```python
from build123d import *

# Parameters (mm, degrees)
SKETCH1_W           = 7.8
SKETCH1_H           = 1
BOSS_EXTRUDE1_DEPTH = 5
SKETCH2_W           = 7.465
SKETCH2_H           = 0.5
CUT_EXTRUDE1_DEPTH  = 0.5
SKETCH3_W           = 14.93
SKETCH3_H           = 0.5
CUT_EXTRUDE2_DEPTH  = 0.5
BOSS_EXTRUDE2_DEPTH = 0.5
SKETCH5_W           = 1
SKETCH5_H           = 2.195949596
BOSS_EXTRUDE3_DEPTH = 7.5
SKETCH6_W           = 0.2
SKETCH6_H           = 0.5
SKETCH6_W_2         = 0.5
SKETCH6_W_3         = 0.413933432
BOSS_EXTRUDE4_DEPTH = 0.5
SKETCH8_W           = 14.93
SKETCH8_H           = 0.5
CUT_EXTRUDE3_DEPTH  = 0.5
SKETCH9_W           = 14.93
SKETCH9_H           = 0.084331677
CUT_EXTRUDE4_DEPTH  = 0.5
SKETCH12_W          = 14.93
SKETCH12_H          = 1.2
CUT_EXTRUDE5_DEPTH  = 0.5


with BuildPart() as part:
    # Sketch1 → Boss-Extrude1 (new body)
    with BuildSketch(Plane(origin=(0, 0, 0), x_dir=(1, 0, 0), z_dir=(0, 1, 0))):
        with Locations((3.9, 15.43)):
            Rectangle(SKETCH1_W, SKETCH1_H)
        Polygon((7.8, 15.93), (8.8, 14.93), (7.8, 14.93), align=None)
        Polygon((7.8, -1), (7.8, 0), (7.8, 14.93), (8.8, 14.93), (8.8, 0), align=None)
        Polygon((-1, 0), (0, 0), (7.8, 0), (7.8, -1), (0, -1), align=None)
        Polygon((0, 15.93), (0, 14.93), (0, 0), (-1, 0), (-1, 14.93), align=None)
    extrude(amount=BOSS_EXTRUDE1_DEPTH)

    # Sketch2 → Cut-Extrude1 (cut)
    with BuildSketch(Plane(origin=(0, 0, 0), x_dir=(0, 0, -1), z_dir=(1, 0, 0))):
        with Locations((11.1975, 0.75)):
            Rectangle(SKETCH2_W, SKETCH2_H)
        with Locations((3.7325, 0.75)):
            Rectangle(SKETCH2_W, SKETCH2_H)
    extrude(amount=-CUT_EXTRUDE1_DEPTH, mode=Mode.SUBTRACT)

    # Sketch3 → Cut-Extrude2 (cut)
    with BuildSketch(Plane.ZY.offset(-7.8)):
        with Locations((-7.465, 0.75)):
            Rectangle(SKETCH3_W, SKETCH3_H)
    extrude(amount=-CUT_EXTRUDE2_DEPTH, mode=Mode.SUBTRACT)

    # Sketch4 → Boss-Extrude2 (add)
    with BuildSketch(Plane(origin=(0, 5, 0), x_dir=(1, 0, 0), z_dir=(0, 1, 0))):
        Polygon((-1, 0), (0, -1), (7.8, -1), (8.8, 0), (8.8, 14.93), (7.8, 15.93), (0, 15.93), (-1, 14.93), align=None)
    extrude(amount=BOSS_EXTRUDE2_DEPTH)

    # Sketch5 → Boss-Extrude3 (add)
    with BuildSketch(Plane.XZ.offset(-5)):
        with Locations((4.4, -12.832025202)):
            Rectangle(SKETCH5_W, SKETCH5_H)
        with Locations((3.4, -12.832025202)):
            Rectangle(SKETCH5_W, SKETCH5_H)
        with Locations((3.4, -10.636075606)):
            Rectangle(SKETCH5_W, SKETCH5_H)
        with Locations((4.4, -10.636075606)):
            Rectangle(SKETCH5_W, SKETCH5_H)
    extrude(amount=BOSS_EXTRUDE3_DEPTH)

    # Sketch6 → Boss-Extrude4 (add)
    with BuildSketch(Plane.XZ.offset(2.5)):
        with Locations((4, -10.984050404)):
            Rectangle(SKETCH6_W, SKETCH6_H)
        with Locations((3.8, -10.984050404)):
            Rectangle(SKETCH6_W, SKETCH6_H)
        with Locations((3.8, -11.484050404)):
            Rectangle(SKETCH6_W, SKETCH6_H)
        with Locations((4, -11.484050404)):
            Rectangle(SKETCH6_W, SKETCH6_H)
        with Locations((4.35, -11.484050404)):
            Rectangle(SKETCH6_W_2, SKETCH6_H)
        with Locations((4.35, -11.984050404)):
            Rectangle(SKETCH6_W_2, SKETCH6_H)
        Polygon((3.9, -11.734050404), (3.7, -11.734050404), (3.7, -12.234050404), (3.986066568, -12.234050404), (4.1, -12.234050404), (4.1, -11.734050404), align=None)
        with Locations((3.493033284, -11.484050404)):
            Rectangle(SKETCH6_W_3, SKETCH6_H)
        with Locations((3.493033284, -11.984050404)):
            Rectangle(SKETCH6_W_3, SKETCH6_H)
        Polygon((3.986066568, -12.234050404), (3.7, -12.234050404), (3.7, -12.768693535), (4.1, -12.768693535), (4.1, -12.234050404), align=None)
    extrude(amount=BOSS_EXTRUDE4_DEPTH)

    # Sketch8 → Cut-Extrude3 (cut)
    with BuildSketch(Plane.ZY.offset(-7.8)):
        with Locations((-7.465, 1.334331677)):
            Rectangle(SKETCH8_W, SKETCH8_H)
    extrude(amount=-CUT_EXTRUDE3_DEPTH, mode=Mode.SUBTRACT)

    # Sketch9 → Cut-Extrude4 (cut)
    with BuildSketch(Plane.ZY.offset(-7.8)):
        with Locations((-7.465, 1.042165838)):
            Rectangle(SKETCH9_W, SKETCH9_H)
    extrude(amount=-CUT_EXTRUDE4_DEPTH, mode=Mode.SUBTRACT)

    # Sketch12 → Cut-Extrude5 (cut)
    with BuildSketch(Plane(origin=(0, 0, 0), x_dir=(0, 0, -1), z_dir=(1, 0, 0))):
        with Locations((7.465, 1.6)):
            Rectangle(SKETCH12_W, SKETCH12_H)
    extrude(amount=-CUT_EXTRUDE5_DEPTH, mode=Mode.SUBTRACT)


solid = part.part
```
Verification items for the finished model (mm, model axes). A direction names the side the tool comes from. Coordinates: 2 decimals unless noted, no trailing zeros. Order: outer loops, then holes, each group sorted by start corner. A loop starts at its lowest first (then second) coordinate and runs counter-clockwise, first axis right, second up. Notation, with made-up numbers: (16.5, 41) -> (59.5, 41) arc R20 cw to (59.5, 57) -> close; hole circle Ø2 at (71, 18.25). An arc over 180 degrees is marked (long way). Put each result on its own line as item: value. Start each with the question number.
1) Tool access check on faces 4 (the flat face through (-0.5, 1, -7)), 5 (the flat face through (4.9, 1, -12)), 6 (the flat face through (-0.49, 2.71, -15.44)). Record the directions out of +Z, -Z, +X, -X, +Y, -Y that give a thin tool (end or side, any length) a straight path to the whole face; none if there is none.
2) Material ranges on L1, parallel to Z at x = 4.5, y = 0.75; L2, parallel to X at y = 2.5, z = -9.75; L3, parallel to Z at x = 0.25, y = 3, recorded low to high.
3) Cross-section at A-A (y = 4). Enter the section's corners in (x, z).
4) Cross-section at D-D (x = 1). Enter the section's corners in (y, z).
5) Go/stop test with flat-tipped pins: pin 1 (2 mm diameter, centred on x = 1.5, y = -0.5, fed in from -Z); pin 2 (0.6 mm diameter, centred on x = 4.5, y = -2.5, fed in from -Z); pin 3 (3 mm diameter, centred on x = 4, z = -6.5, fed in from -Y); pin 4 (0.6 mm diameter, centred on x = 8, z = -11, fed in from -Y). Record where each tip stops, or that it passes through.
6) Cross-section at B-B (z = -9). Enter the section's corners in (x, y).
7) Cross-section at C-C (y = 2). Enter the section's corners in (x, z), plus the area to 3 significant figures.
8) Release check for a two-part mould opening along Y. For faces 1 (the flat face through (8, 0, -7)), 2 (the flat face through (8.3, 1, -8)), 3 (the flat face through (4, 3, 1)) record: pulls with the +Y half, pulls with the -Y half, needs draft (parallel to the pull), parting line crosses it, or undercut.
Geometry check:
1. face 4: none
1. face 5: -Y
1. face 6: -Z, -X, +Y, -Y
2. L1: z = -15.93 to -14.93, -13.93 to -9.54, 0 to 1
2. L2: x = -1 to 0, 2.9 to 4.9, 7.8 to 8.8
2. L3: z = -15.93 to -14.93, 0 to 1
3. outline: (-1, -14.93) -> (0, -15.93) -> (7.8, -15.93) -> (8.8, -14.93) -> (8.8, 0) -> (7.8, 1) -> (0, 1) -> (-1, 0) -> close; (2.9, -13.93) -> (4.9, -13.93) -> (4.9, -9.54) -> (2.9, -9.54) -> close; hole (0, -14.93) -> (7.8, -14.93) -> (7.8, 0) -> (0, 0) -> close
4. outline: (0, -15.93) -> (5.5, -15.93) -> (5.5, 1) -> (0, 1) -> (0, 0) -> (5, 0) -> (5, -14.93) -> (0, -14.93) -> close
5. pin 1: stops at z = -15.93
5. pin 2: stops at z = -13.93
5. pin 3: stops at y = 5
5. pin 4: stops at y = 0
6. outline: (-1, 0) -> (0, 0) -> (0, 0.5) -> (-0.5, 0.5) -> (-0.5, 2.2) -> (0, 2.2) -> (0, 5) -> (7.8, 5) -> (7.8, 1.58) -> (8.3, 1.58) -> (8.3, 0.5) -> (7.8, 0.5) -> (7.8, 0) -> (8.8, 0) -> (8.8, 5.5) -> (-1, 5.5) -> close
7. outline: (-1, -14.93) -> (0, -15.93) -> (7.8, -15.93) -> (8.8, -14.93) -> (8.8, 0) -> (7.8, 1) -> (0, 1) -> (-1, 0) -> close; (2.9, -13.93) -> (4.9, -13.93) -> (4.9, -9.54) -> (2.9, -9.54) -> close; hole (-0.5, -14.93) -> (7.8, -14.93) -> (7.8, 0) -> (-0.5, 0) -> close
7. area: 48.8 mm^2
8. face 1: pulls with the -Y half
8. face 2: undercut
8. face 3: needs draft
